Read the model definition and answer for the solid it produces. Units are mm, in the model's axes. A direction names the side the tool comes from. Coordinates: 2 decimals unless noted, no trailing zeros. Write each loop counter-clockwise with the first axis right and the second up, starting at its lowest first coordinate (ties: lowest second). Pieces come first, ordered by that corner, then holes. Notation, with made-up numbers: (60, 76) -> (114, 76) arc R28 ccw to (114, 107) -> close; hole circle Ø4 at (17.25, 26). An arc over 180 degrees is marked (long way). Use CSV: the item, a comma, the result in double quotes. Start each with the question number.
from build123d import *

# Parameters (mm, degrees)
SKETCH1_W               = 20
SKETCH1_H               = 28
SKETCH1_R               = 1.275
BOSS_EXTRUDE1_DEPTH     = 2.1
SKETCH1_3_W             = 8.5
SKETCH1_3_H             = 25
BOSS_EXTRUDE2_DEPTH     = 24.1
CUT_EXTRUDE1_DEPTH      = 5
CUT_EXTRUDE2_DEPTH      = 46.486921197
CUT_EXTRUDE2_DEPTH_BACK = 46.486921197
CUT_EXTRUDE3_DEPTH      = 17
CUT_EXTRUDE4_REACH      = 48.659
FILLET1_R               = 1


with BuildPart() as part:
    # Sketch1 → Boss-Extrude1 (new body)
    with BuildSketch(Plane.XY):
        with Locations((10, 14)):
            Rectangle(SKETCH1_W, SKETCH1_H)
        with Locations((10, 8)):
            Circle(SKETCH1_R, mode=Mode.SUBTRACT)
        with Locations((13, 5)):
            Circle(SKETCH1_R, mode=Mode.SUBTRACT)
        with Locations((16, 14)):
            Circle(SKETCH1_R, mode=Mode.SUBTRACT)
        with Locations((4, 14)):
            Circle(SKETCH1_R, mode=Mode.SUBTRACT)
        with Locations((7, 23)):
            Circle(SKETCH1_R, mode=Mode.SUBTRACT)
        with Locations((10, 20)):
            Circle(SKETCH1_R, mode=Mode.SUBTRACT)
        with Locations((13, 23)):
            Circle(SKETCH1_R, mode=Mode.SUBTRACT)
        with Locations((7, 5)):
            Circle(SKETCH1_R, mode=Mode.SUBTRACT)
    extrude(amount=-BOSS_EXTRUDE1_DEPTH)

    # Sketch1_3 → Boss-Extrude2 (add)
    with BuildSketch(Plane.XY):
        with Locations((24.25, 13.5)):
            Rectangle(SKETCH1_3_W, SKETCH1_3_H)
    extrude(amount=-BOSS_EXTRUDE2_DEPTH)

    # Sketch2 → Cut-Extrude1 (cut)
    with BuildSketch(Plane(origin=(28.5, 0, 0), x_dir=(0, 0, -1), z_dir=(1, 0, 0))):
        with BuildLine():
            Line((0, 23), (6, 23))
            ThreePointArc((6, 23), (8.828427125, 21.828427125), (10, 19))
            Line((10, 19), (10, 16))
            ThreePointArc((10, 16), (8.828427125, 13.171572875), (6, 12))
            Line((6, 12), (0, 9.797))
            Line((0, 9.797), (0, 23))
        make_face()
    extrude(amount=-CUT_EXTRUDE1_DEPTH, mode=Mode.SUBTRACT)

    # Sketch3 → Cut-Extrude2 (cut, two sides: drawn at the far end of the back side and taken through both)
    with BuildSketch(Plane(origin=(0, 26, 0), x_dir=(1, 0, 0), z_dir=(0, 1, 0)).offset(-CUT_EXTRUDE2_DEPTH_BACK)):
        with BuildLine():
            Line((24.75, 20.85), (24.25, 20.85))
            ThreePointArc((24.25, 20.85), (22.835786438, 20.264213562), (22.25, 18.85))
            Line((22.25, 18.85), (22.25, 10.1))
            ThreePointArc((22.25, 10.1), (22.835786438, 8.685786438), (24.25, 8.1))
            Line((24.25, 8.1), (24.75, 8.1))
            ThreePointArc((24.75, 8.1), (26.164213562, 8.685786438), (26.75, 10.1))
            Line((26.75, 10.1), (26.75, 18.85))
            ThreePointArc((26.75, 18.85), (26.164213562, 20.264213562), (24.75, 20.85))
        make_face()
    extrude(amount=CUT_EXTRUDE2_DEPTH + CUT_EXTRUDE2_DEPTH_BACK, mode=Mode.SUBTRACT)

    # Sketch4 → Cut-Extrude3 (cut)
    with BuildSketch(Plane(origin=(0, 0, -24.1), x_dir=(-1, 0, 0), z_dir=(0, 0, -1))):
        with BuildLine():
            Line((-20, 11.5), (-25, 11.5))
            ThreePointArc((-25, 11.5), (-25.707106781, 11.792893219), (-26, 12.5))
            Line((-26, 12.5), (-26, 21.5))
            ThreePointArc((-26, 21.5), (-25.707106781, 22.207106781), (-25, 22.5))
            Line((-25, 22.5), (-20, 22.5))
            Line((-20, 22.5), (-20, 11.5))
        make_face()
    extrude(amount=-CUT_EXTRUDE3_DEPTH, mode=Mode.SUBTRACT)

    # Sketch6 → Cut-Extrude4 (cut, up to next)
    with BuildSketch(Plane(origin=(28.5, 0, 0), x_dir=(0, 0, -1), z_dir=(1, 0, 0)), mode=Mode.PRIVATE) as cut_extrude4_sk1:
        Polygon((2.1, 1), (24.1, 1), (24.1, 8), (7.973697418, 8), align=None)
    cut_extrude4_tool1 = extrude(cut_extrude4_sk1.sketch, amount=-CUT_EXTRUDE4_REACH, mode=Mode.PRIVATE) & part.part
    add(cut_extrude4_tool1.solids().sort_by_distance((28.5, 4.320265, -14.493016))[0], mode=Mode.SUBTRACT)

    # Fillet1
    fillet1_edges = [part.edges().sort_by_distance(p)[0] for p in [
        (28.5, 8, -16.036848709),
        (28.5, 26, -12.05),
    ]]
    fillet(fillet1_edges, radius=FILLET1_R)


solid = part.part
1) Section C-C, the plane x = 7 is taken. Give the vertices of the cut face in (y, z) (3 decimals).
2) Section D-D, the plane y = 20 is taken. Give the vertices of the cut face in (x, z) (3 decimals), plus the area to 3 significant figures.
3) Each of these flat-tipped pins is pushed along its axis until it touches: pin 1 (3 mm diameter, centred on x = 7, y = 5, fed in from -Z); pin 2 (8 mm diameter, centred on x = 22, z = -6.5, fed in from +Y); pin 3 (1.5 mm diameter, centred on y = 14.5, z = -9, fed in from -X); pin 4 (1 mm diameter, centred on x = 19, z = -6.5, fed in from -Y). Where does it stop, or does it pass through?
4) Section B-B, the plane x = 16 is taken. Give the vertices of the cut face in (y, z) (3 decimals), plus the area to 3 significant figures.
5) Section A-A, the plane z = -10.5 is taken. Give the vertices of the cut face in (x, y), plus the area to 3 significant figures.
6) Which of the six approach directions +Z, -Z, +X, -X, +Y, -Y give full straight-line access (tool end or side, diameter ignored) to faces 5 (the face through (24, 1, -1)), 6 (the face through (22, 8, -18)), 7 (the face through (22.82, 9.73, -8.7)), 8 (the face through (22, 22.5, -16))?
7) The mould has two halves that part along X. Classify faces 1 (the face through (22.85, 9.73, -20.28)), 2 (the face through (22, 26, -12)), 3 (the face through (26, 17, -22)), 4 (the face through (26.4, 16.87, -19.98)): pulls with the +X half, pulls with the -X half, needs draft (parallel to the pull), parting line crosses it, or undercut.
8) Find the intervals of material crossed by line 1 along Y through (x, z) = (7, -1.3) (3 decimals); line 2 along Y through (x, z) = (10, -0.8) (3 decimals); line 3 along Y through (x, z) = (4, -0.7) (3 decimals), in increasing order.
The answers:
1,outline,"(0, -2.1) -> (3.725, -2.1) -> (3.725, 0) -> (0, 0) -> close; (6.275, -2.1) -> (21.725, -2.1) -> (21.725, 0) -> (6.275, 0) -> close; (24.275, -2.1) -> (28, -2.1) -> (28, 0) -> (24.275, 0) -> close"
2,outline,"(0, -2.1) -> (8.725, -2.1) -> (8.725, 0) -> (0, 0) -> close; (11.275, -2.1) -> (20, -2.1) -> (20, -7.1) -> (23.5, -7.1) -> (23.5, 0) -> (11.275, 0) -> close; (26, -24.1) -> (28.5, -24.1) -> (28.5, -9.873) -> (26.737, -9.873) arc R2 cw to (26.75, -10.1) -> (26.75, -18.85) arc R2 cw to (26, -20.411) -> close"
2,area,"89.5 mm^2"
3,pin 1,"stops at z = -2.1"
3,pin 2,"stops at y = 26"
3,pin 3,"stops at x = 26.61"
3,pin 4,"passes through"
4,outline,"(0, -2.1) -> (12.725, -2.1) -> (12.725, 0) -> (0, 0) -> close; (15.275, -2.1) -> (28, -2.1) -> (28, 0) -> (15.275, 0) -> close"
4,area,"53.4 mm^2"
5,outline,"(20, 8) -> (22.25, 8) -> (22.25, 11.5) -> (20, 11.5) -> close; (20, 22.5) -> (22.25, 22.5) -> (22.25, 26) -> (20, 26) -> close; (26.75, 8) -> (27.5, 8) arc R1 ccw to (28.5, 9) -> (28.5, 25) arc R1 ccw to (27.5, 26) -> (26.75, 26) -> close"
5,area,"46.8 mm^2"
6,face 5,"+Z, -Z, +X, -Y"
6,face 6,"-Z, +X, -X, -Y"
6,face 7,"+Y, -Y"
6,face 8,"-Z, -X"
7,face 1,"undercut"
7,face 2,"needs draft"
7,face 3,"pulls with the -X half"
7,face 4,"undercut"
8,line 1,"y = 0 to 3.725, 6.275 to 21.725, 24.275 to 28"
8,line 2,"y = 0 to 6.725, 9.275 to 18.725, 21.275 to 28"
8,line 3,"y = 0 to 12.725, 15.275 to 28"
